Check sheet for the modelled part. Datum: model origin and axes. Units: mm. Coordinates: 2 decimals unless noted, no trailing zeros. Write each loop counter-clockwise with the first axis right and the second up, starting at its lowest first coordinate (ties: lowest second). Pieces come first, ordered by that corner, then holes. Notation, with made-up numbers: M -17,10.5 L 28,10.5 A20 cw 28,32.5 Z; hole C 33,-23.75 d1. An arc over 180 degrees is marked long. Answer as CSV lines item,"result".
from build123d import *

# Parameters (mm, degrees)
SKETCH1_W            = 200
SKETCH1_H            = 30
BASE_DEPTH           = 6.35
WEDGECUT_REACH       = 202.662
SKETCH3_W            = 19.745999878
SKETCH3_H            = 6.604
HINGE_CUTOUT_DEPTH   = 0.635
HINGE_HOLE_CUT_REACH = 103.28
SKETCH4_R            = 1.8034
SKETCH5_W            = 5.05
SKETCH5_H            = 5.05
HINGE_NUT_CUT_DEPTH  = 2


with BuildPart() as part:
    # Sketch1 → Base (new body)
    with BuildSketch(Plane(origin=(0, 0, 0), x_dir=(1, 0, 0), z_dir=(0, 1, 0))):
        Rectangle(SKETCH1_W, SKETCH1_H)
    extrude(amount=BASE_DEPTH)

    # Sketch2 → WedgeCut (cut, up to next)
    with BuildSketch(Plane(origin=(100, 0, 0), x_dir=(0, 0, -1), z_dir=(1, 0, 0)), mode=Mode.PRIVATE) as wedgecut_sk1:
        Polygon((-15, 0), (-6.907470508, 0), (8.342084542, 5.407501552), (8.007874016, 6.35), (-15, 6.35), align=None)
    wedgecut_tool1 = extrude(wedgecut_sk1.sketch, amount=-WEDGECUT_REACH, mode=Mode.PRIVATE) & part.part
    add(wedgecut_tool1.solids().sort_by_distance((100, 3.70048, 5.888491))[0], mode=Mode.SUBTRACT)

    # Sketch3 → Hinge Cutout (cut)
    with BuildSketch(Plane(origin=(0, 6.35, 0), x_dir=(1, 0, 0), z_dir=(0, 1, 0))):
        with Locations((-80.127000061, 11.698)):
            Rectangle(SKETCH3_W, SKETCH3_H)
        with Locations((80.127000061, 11.698)):
            Rectangle(SKETCH3_W, SKETCH3_H)
    extrude(amount=-HINGE_CUTOUT_DEPTH, mode=Mode.SUBTRACT)

    # Sketch4 → Hinge Hole Cut (cut, up to next)
    with BuildSketch(Plane(origin=(0, 5.715, 0), x_dir=(1, 0, 0), z_dir=(0, 1, 0)), mode=Mode.PRIVATE) as hinge_hole_cut_sk1:
        with Locations(Location((74.564400061, 11.825, 0), (0, 0, 270))):
            Circle(SKETCH4_R)
    hinge_hole_cut_tool1 = extrude(hinge_hole_cut_sk1.sketch, amount=-HINGE_HOLE_CUT_REACH, mode=Mode.PRIVATE) & part.part
    # Sketch4 → Hinge Hole Cut (cut, up to next)
    with BuildSketch(Plane(origin=(0, 5.715, 0), x_dir=(1, 0, 0), z_dir=(0, 1, 0)), mode=Mode.PRIVATE) as hinge_hole_cut_sk2:
        with Locations(Location((85.689600061, 11.825, 0), (0, 0, 270))):
            Circle(SKETCH4_R)
    hinge_hole_cut_tool2 = extrude(hinge_hole_cut_sk2.sketch, amount=-HINGE_HOLE_CUT_REACH, mode=Mode.PRIVATE) & part.part
    hinge_hole_cut_1 = hinge_hole_cut_tool1.solids().sort_by_distance((74.5644, 5.715, -11.825))[0]
    add(hinge_hole_cut_1, mode=Mode.SUBTRACT)
    hinge_hole_cut_2 = hinge_hole_cut_tool2.solids().sort_by_distance((85.6896, 5.715, -11.825))[0]
    add(hinge_hole_cut_2, mode=Mode.SUBTRACT)
    hinge_hole_cut = hinge_hole_cut_1 + hinge_hole_cut_2  # Hinge Hole Cut as one shape, for the pattern or mirror that repeats it

    # Sketch5 → Hinge Nut Cut (cut)
    with BuildSketch(Plane.XZ):
        with Locations((74.564400061, -11.825)):
            Rectangle(SKETCH5_W, SKETCH5_H)
        with Locations((85.689600061, -11.825)):
            Rectangle(SKETCH5_W, SKETCH5_H)
    hinge_nut_cut = extrude(amount=-HINGE_NUT_CUT_DEPTH, mode=Mode.SUBTRACT)

    # Hinge Hole Mirror: Hinge Hole Cut, Hinge Nut Cut across plane
    add(hinge_hole_cut.mirror(Plane(origin=(0, 0, 0), x_dir=(0, 0, 1), z_dir=(1, 0, 0))), mode=Mode.SUBTRACT)
    add(hinge_nut_cut.mirror(Plane(origin=(0, 0, 0), x_dir=(0, 0, 1), z_dir=(1, 0, 0))), mode=Mode.SUBTRACT)


solid = part.part
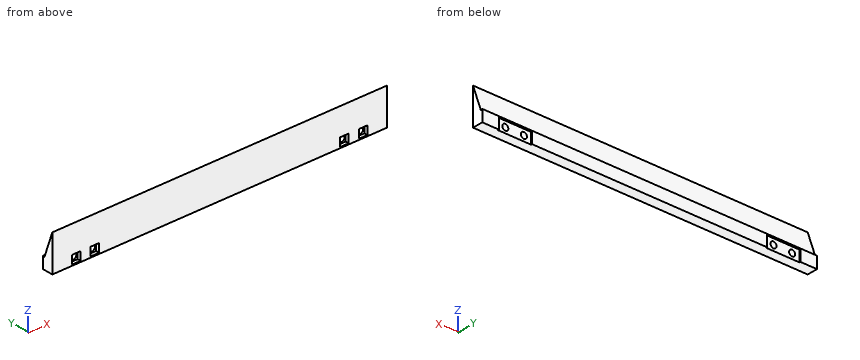
1) Thickness scan on line 1 along X through (y, z) = (3, -10.25); line 2 along Y through (x, z) = (-79.5, -5); line 3 along Z through (x, y) = (-19.5, 5.75). Record the ranges inside material, lowest first.
Answer key:
line 1,"x = -100 to -86.57, -84.81 to -75.44, -73.69 to 73.69, 75.44 to 84.81, 86.57 to 100"
line 2,"y = 0 to 4.22"
line 3,"z = -15 to -8.22"
2) Depth check by flat-ended pin: P1, Ø2.5, axis at x = 85.5, z = -13, coming from the -Y side; P2, Ø4, axis at x = -56.5, z = -2, coming from the +Y side; P3, Ø3.5, axis at x = 83.5, z = -11, coming from the +Y side (3 decimals). Enter the tip coordinate at first touch or a pass-through.
Answer key:
P1,"stops at y = 2"
P2,"stops at y = 3.87"
P3,"stops at y = 5.715"
3) Section check A-A, the plane y = 3.75. Record the boundary of the cut face in (x, z) (3 decimals).
Answer key:
outline,"M -100,-15 L 100,-15 L 100,-3.668 L -100,-3.668 Z; hole C -85.69,-11.825 d3.607; hole C -74.564,-11.825 d3.607; hole C 74.564,-11.825 d3.607; hole C 85.69,-11.825 d3.607"
4) Section check C-C, the plane z = -3.75. Record the boundary of the cut face in (x, y).
Answer key:
outline,"M -100,0 L 100,0 L 100,3.78 L -100,3.78 Z"
5) Section check B-B, the plane x = 4.5. Record the boundary of the cut face in (y, z).
Answer key:
outline,"M 0,-15 L 6.35,-15 L 6.35,-8.01 L 5.41,-8.34 L 0,6.91 Z"
